Design review of the part built by this model. Coordinates are the model's own, in mm. Face numbers are marked on the shaded views. A direction names the side the tool comes from. Coordinates: 2 decimals unless noted, no trailing zeros. Loops run counter-clockwise (first coordinate to the right, second up) from the corner with the lowest first, then second, coordinate; pieces in that order, holes last. Notation, with made-up numbers: (66.5, 31.25) -> (106.5, 31.25) arc R11 ccw to (106.5, 51.25) -> close; hole circle Ø1 at (22.25, -12). An arc over 180 degrees is marked (long way). Answer as a JSON object with one key per item and string values.
```python
from build123d import *

# Parameters (mm, degrees)
F0_R        = 1.5
F1_DEPTH    = 3
F2_W        = 3
F2_H        = 35
F3_DEPTH    = 25
F4_W        = 13
F4_H        = 24
F4_R        = 0.875
F5_DEPTH    = 27.001
F6_W        = 20
F6_H        = 3
F7_DEPTH    = 23
F8_T4_DEPTH = 121.2974174464


# Not quite as in the source:
# - a fillet or chamfer that OpenCascade refuses, or shapes differently, is made with other operations: its cross-section is extruded or revolved along the edge and cut away or added
# - a feature of the source that left no trace in its solid (it failed there, or was rolled back) is left out


with BuildPart() as f1:
    # F0 (on Front) → F1 (new body)
    with BuildSketch(Plane.XZ):
        Polygon((-19.1084720148, 23.034380586), (-19.1084720148, 0), (25.8915279852, 0), (25.8915279852, 32), (22.8915279852, 35), (-7.1428526009, 35), align=None)
        with Locations((-14.1084720148, 3)):
            Circle(F0_R, mode=Mode.SUBTRACT)
        with Locations((20.8915279852, 26)):
            Circle(F0_R, mode=Mode.SUBTRACT)
    extrude(amount=F1_DEPTH)

    # F2 (on face) → F3 (join)
    with BuildSketch(Plane.XZ.offset(3)):
        with Locations((0.3915279852, 17.5)):
            Rectangle(F2_W, F2_H)
    extrude(amount=F3_DEPTH)

    # F4 (on face) → F5 (cut, through all)
    with BuildSketch(Plane(origin=(-1.1084720148, 0, 0), x_dir=(0, -1, 0), z_dir=(-1, 0, 0))):
        with Locations((15.5, 17.5)):
            Rectangle(F4_W, F4_H)
        with Locations((15.5, 32)):
            Circle(F4_R)
        with Locations((15.5, 3)):
            Circle(F4_R)
    extrude(amount=-F5_DEPTH, mode=Mode.SUBTRACT)

    # F6 (on face) → F7 (join)
    with BuildSketch(Plane.XZ.offset(3)):
        with Locations((11.8915279852, 33)):
            Rectangle(F6_W, F6_H)
        with Locations((11.8915279852, 2)):
            Rectangle(F6_W, F6_H)
    extrude(amount=F7_DEPTH)

    # F8: chamfer of 23 on 1 edges, made by hand


with BuildPart() as f8_tool2:
    # F8_s3 → F8_t4 (new body)
    with BuildSketch(Plane.XY.offset(-58.6487087232)):
        Polygon((21.8915279852, -3), (-1.1084720148, -26), (21.8915279852, -26), align=None)
    extrude(amount=F8_T4_DEPTH)

    split(bisect_by=Plane.XZ.offset(3), keep=Keep.TOP)

    split(bisect_by=Plane.YZ.offset(1.8915279852), keep=Keep.TOP)


with BuildPart() as f1_1:
    add(f1.part)

    # F8_t1: cut F8_tool2
    add(f8_tool2.part, mode=Mode.SUBTRACT)


solid = f1_1.part
```
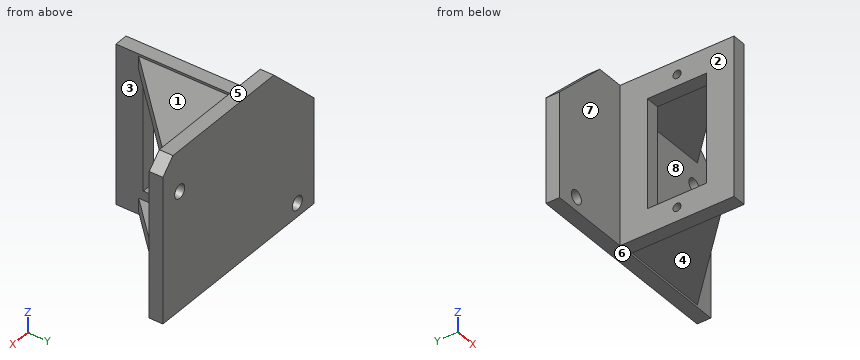
1) The part is to be moulded in two halves that separate along Z. For the marked faces 5, 6, 7 and 8, say which applies: pulls with the +Z half, pulls with the -Z half, needs draft (parallel to the pull), parting line crosses it, or undercut.
Completed:
{"face 5": "pulls with the +Z half", "face 6": "pulls with the -Z half", "face 7": "needs draft", "face 8": "undercut"}
2) Add section A-A, the plane z = 8.5. Give the boundary of the cut face in (x, y), and give its area (3 significant figures).
Completed:
{"outline": "(-19.11, -3) -> (-1.11, -3) -> (-1.11, -9) -> (1.89, -9) -> (1.89, -3) -> (25.89, -3) -> (25.89, 0) -> (-19.11, 0) -> close; (-1.11, -28) -> (1.89, -28) -> (1.89, -22) -> (-1.11, -22) -> close", "area": "171 mm²"}
3) Add section C-C, the plane x = -13.5. Give the boundary of the cut face in (y, z), and give its area (3 significant figures).
Completed:
{"outline": "(-3, 0) -> (0, 0) -> (0, 1.63) -> (-3, 1.63) -> close; (-3, 4.37) -> (0, 4.37) -> (0, 28.64) -> (-3, 28.64) -> close", "area": "77.7 mm²"}
4) Add section B-B, the plane y = -2. Give the boundary of the cut face in (x, z).
Completed:
{"outline": "(-19.11, 0) -> (25.89, 0) -> (25.89, 32) -> (22.89, 35) -> (-7.14, 35) -> (-19.11, 23.03) -> close; hole circle Ø3 at (-14.11, 3); hole circle Ø3 at (20.89, 26)"}
5) Clearance check with flat-ended pins moving along their axes: pin 1 Ø3 at (x, z) = (-3.5, 31) entering from -Y; pin 2 Ø2.5 at (y, z) = (-15.5, 3) entering from +X; pin 3 Ø1.5 at (x, y) = (18.5, -9) entering from -Z; pin 4 Ø6 at (y, z) = (-10.5, 6) entering from +X. State where each tip first meets the part, or that it passes through.
Completed:
{"pin 1": "y = -3", "pin 2": "x = 10.64", "pin 3": "through", "pin 4": "x = 16.05"}
6) Add section D-D, the plane y = -11.5. Give the boundary of the cut face in (x, z).
Completed:
{"outline": "(-1.11, 0) -> (1.89, 0) -> (1.89, 0.5) -> (13.39, 0.5) -> (13.39, 3.5) -> (1.89, 3.5) -> (1.89, 5.5) -> (-1.11, 5.5) -> close; (-1.11, 29.5) -> (1.89, 29.5) -> (1.89, 31.5) -> (13.39, 31.5) -> (13.39, 34.5) -> (1.89, 34.5) -> (1.89, 35) -> (-1.11, 35) -> close"}
7) For the marked faces 1, 2, 3 and 4, list the 3-axis set-ups (+Z, -Z, +X, -X, +Y, -Y) from which the entire face can be reached by the end or side of a thin tool; tool diameter is ignored.
Completed:
{"face 1": "+Z, +X, -Y", "face 2": "+Z, -Z, -X, -Y", "face 3": "+X, -Y", "face 4": "-Z, +X, -Y"}
8) Wall thickness on probe 1 along Z at (x, y) = (0.65, -15.5) (3 decimals); probe 2 along Z at (x, y) = (12, -4.25); probe 3 along Y at (x, z) = (-1, 17): over which ranges is each line inside the solid? List them lowest first.
Completed:
{"probe 1": "0 to 2.125, 3.875 to 5.5, 29.5 to 31.125, 32.875 to 35", "probe 2": "0.5 to 3.5, 31.5 to 34.5", "probe 3": "-28 to -22, -9 to 0"}
